Here's how the part is built. I have some questions about the finished solid (model axes, mm). Coordinates: 2 decimals unless noted, no trailing zeros. Loops run counter-clockwise (first coordinate to the right, second up) from the corner with the lowest first, then second, coordinate; pieces in that order, holes last. Notation, with made-up numbers: (14, 0) - (44, 0) arc R13 cw to (44, 24) - close; hole circle Ø6 at (-29.75, 20.5). An arc over 180 degrees is marked (long way). Use a Markdown table: item, result.
```python
from build123d import *

# Parameters (mm, degrees)
SKETCH1_W           = 228.6
SKETCH1_H           = 139.7
SKETCH1_R           = 1.778
BOSS_EXTRUDE1_DEPTH = 3.175
SKETCH3_R           = 1.524
CUT_EXTRUDE1_DEPTH  = 4.175
SKETCH4_R           = 1.5875
CUT_EXTRUDE2_DEPTH  = 4.175
SKETCH5_R           = 1.5875
CUT_EXTRUDE3_DEPTH  = 4.175
CUT_EXTRUDE4_DEPTH  = 4.175
FILLET1_R           = 2.54
SKETCH7_R           = 1.5875
CUT_EXTRUDE5_DEPTH  = 4.175


with BuildPart() as part:
    # Sketch1 → Boss-Extrude1 (new body)
    with BuildSketch(Plane(origin=(0, 0, 0), x_dir=(1, 0, 0), z_dir=(0, 1, 0))):
        with Locations((114.3, 69.85)):
            Rectangle(SKETCH1_W, SKETCH1_H)
        with Locations((86.36, 127)):
            Circle(SKETCH1_R, mode=Mode.SUBTRACT)
        with Locations((142.24, 127)):
            Circle(SKETCH1_R, mode=Mode.SUBTRACT)
        with Locations((86.36, 87.63)):
            Circle(SKETCH1_R, mode=Mode.SUBTRACT)
        with Locations((142.24, 87.63)):
            Circle(SKETCH1_R, mode=Mode.SUBTRACT)
    extrude(amount=BOSS_EXTRUDE1_DEPTH)

    # Sketch3 → Cut-Extrude1 (cut, through all)
    with BuildSketch(Plane(origin=(0, 3.175, 0), x_dir=(1, 0, 0), z_dir=(0, 1, 0))):
        with Locations((69.85, 70.485)):
            Circle(SKETCH3_R)
        with Locations((158.75, 70.485)):
            Circle(SKETCH3_R)
        with Locations((158.75, 9.525)):
            Circle(SKETCH3_R)
        with Locations((69.85, 9.525)):
            Circle(SKETCH3_R)
    extrude(amount=-CUT_EXTRUDE1_DEPTH, mode=Mode.SUBTRACT)

    # Sketch4 → Cut-Extrude2 (cut, through all)
    with BuildSketch(Plane(origin=(0, 3.175, 0), x_dir=(1, 0, 0), z_dir=(0, 1, 0))):
        with Locations((171.0182, 21.94814)):
            Circle(SKETCH4_R)
        with Locations((186.2582, 72.74814)):
            Circle(SKETCH4_R)
        with Locations((214.1982, 72.74814)):
            Circle(SKETCH4_R)
        with Locations((219.2782, 20.67814)):
            Circle(SKETCH4_R)
    extrude(amount=-CUT_EXTRUDE2_DEPTH, mode=Mode.SUBTRACT)

    # Sketch5 → Cut-Extrude3 (cut, through all)
    with BuildSketch(Plane(origin=(0, 3.175, 0), x_dir=(1, 0, 0), z_dir=(0, 1, 0))):
        with Locations((14.605, 71.755)):
            Circle(SKETCH5_R)
        with Locations((55.245, 71.755)):
            Circle(SKETCH5_R)
        with Locations((55.245, 8.89)):
            Circle(SKETCH5_R)
        with Locations((14.605, 8.89)):
            Circle(SKETCH5_R)
    extrude(amount=-CUT_EXTRUDE3_DEPTH, mode=Mode.SUBTRACT)

    # Sketch6 → Cut-Extrude4 (cut, through all)
    with BuildSketch(Plane(origin=(0, 3.175, 0), x_dir=(1, 0, 0), z_dir=(0, 1, 0))):
        Polygon((228.6, 79.248), (152.4, 139.7), (228.6, 139.7), align=None)
        Polygon((76.2, 139.7), (0, 139.7), (0, 79.248), align=None)
    extrude(amount=-CUT_EXTRUDE4_DEPTH, mode=Mode.SUBTRACT)

    # Fillet1
    fillet1_edges = [part.edges().sort_by_distance(p)[0] for p in [
        (228.6, 1.5875, 0),
        (0, 1.5875, 0),
        (228.6, 1.5875, -79.248),
        (152.4, 1.5875, -139.7),
        (76.2, 1.5875, -139.7),
        (0, 1.5875, -79.248),
    ]]
    fillet(fillet1_edges, radius=FILLET1_R)

    # Sketch7 → Cut-Extrude5 (cut, through all)
    with BuildSketch(Plane(origin=(0, 3.175, 0), x_dir=(1, 0, 0), z_dir=(0, 1, 0))):
        with Locations((220.98, 7.62)):
            Circle(SKETCH7_R)
        with Locations((149.744486069, 132.08)):
            Circle(SKETCH7_R)
        with Locations((7.62, 7.62)):
            Circle(SKETCH7_R)
        with Locations((78.855513931, 132.08)):
            Circle(SKETCH7_R)
    extrude(amount=-CUT_EXTRUDE5_DEPTH, mode=Mode.SUBTRACT)


solid = part.part
```
Q1. I want a section at A-A, the plane y = 2.45. Give the number of separate pieces and of enclosed holes in the cut face, then the cut area to 3 significant figures.
Check values:
| item | result |
|---|---|
| separate pieces | 1 |
| enclosed holes | 20 |
| area | 27,200 mm^2 |
Q2. I want a section at C-C, the plane z = -95. Write out the boundary of the cut face in (x, y) (3 decimals), then the cut area to 3 significant figures.
Check values:
| item | result |
|---|---|
| outline | (19.855, 0) - (208.745, 0) - (208.745, 3.175) - (19.855, 3.175) - close |
| area | 600 mm^2 |
Q3. Please list where these lines run through material, in increasing order: L1, parallel to X at y = 1.6, z = -132.08; L2, parallel to X at y = 1.05, z = -20.5; L3, parallel to Z at x = 158.75, y = 2.1. Write a range as from..to.
Check values:
| item | result |
|---|---|
| L1 | 66.59..77.27, 80.44..148.16, 151.33..162.01 |
| L2 | 0..170.37, 171.67..217.7, 220.86..228.6 |
| L3 | -134.66..-72.01, -68.96..-11.05, -8..0 |
Q4. I want a section at B-B, the plane x = 61. Write out the boundary of the cut face in (y, z) (3 decimals).
Check values:
| item | result |
|---|---|
| outline | (0, -127.641) - (3.175, -127.641) - (3.175, 0) - (0, 0) - close |
